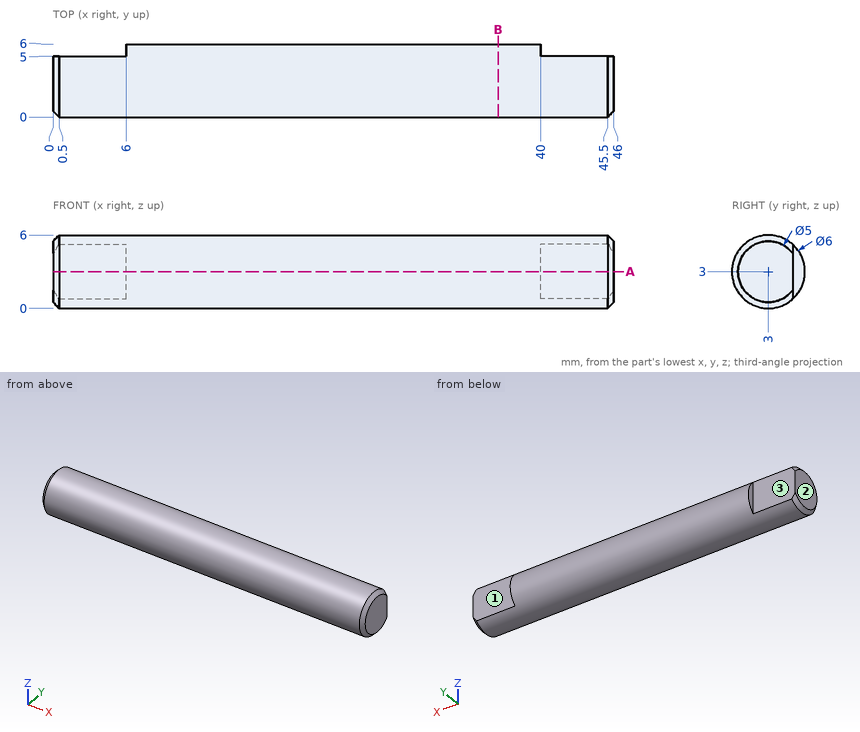
Geometry: see drawing. Coordinates: mm, zero at the bounding-box minimum. A direction names the side the tool comes from. Give positions to 0.01 mm unless a question says otherwise; leave off trailing zeros. Write each loop counter-clockwise with the first axis right and the second up, starting at its lowest first coordinate (ties: lowest second). Pieces come first, ordered by that corner, then holes. Notation, with made-up numbers: M 33,86 L 58,86 A10 cw 58,92 Z; hole C -12.5,65.5 d3. An arc over 180 degrees is marked long. Return JSON: item names as keys, results as strings. Group by question number.
1) Cut plane A-A, the plane z = 3. Output: boundary loops of the cut face in (x, y).
2) Cut plane B-B, the plane x = 36.5. Output: boundary loops of the cut face in (y, z), then the cut area to 3 significant figures.
3) Ray query, L1, parallel to X at y = 2, z = 5.3; L2, parallel to Y at x = 28, z = 2.9; L3, parallel to Y at x = 6.5, z = 1. Return the intervals inside material, ascending.
4) Set-up query: the marked faces 1, 2 and 3. Return all of +Z, -Z, +X, -X, +Y, -Y with unobstructed straight access to the full face (end or side cutting, diameter ignored); none if empty.
5) First-contact query: pin 1 Ø3.5 at (x, z) = (2.5, 2.5) entering from +Y; pin 2 Ø1 at (x, y) = (7, 1) entering from -Z; pin 3 Ø1.5 at (y, z) = (4.5, 1.5) entering from -X; pin 4 Ø1.5 at (x, z) = (29, 5) entering from -Y. Flat tips, straight axial feed; report the tip coordinate or a pass-through.
Data:
{
 "1": {"outline": "M 0,0.5 L 0.5,0 L 45.5,0 L 46,0.5 L 46,5 L 40,5 L 40,6 L 6,6 L 6,5 L 0,5 Z"},
 "2": {"outline": "C 3,3 d6", "area": "28.3 mm²"},
 "3": {"L1": "x = 0.01 to 45.99", "L2": "y = 0 to 6", "L3": "y = 0.76 to 5.24"},
 "4": {"face 1": "+Z, -Z, +X, +Y", "face 2": "+Z, -Z, -X, +Y, -Y", "face 3": "+Z, -Z, -X, +Y"},
 "5": {"pin 1": "stops at y = 5", "pin 2": "stops at z = 0.4", "pin 3": "stops at x = 0", "pin 4": "stops at y = 0.27"}
}
